Geometry: final body of the model. Coordinates: model frame, mm. A direction names the side the tool comes from. Give positions to 0.01 mm unless a question says otherwise; leave off trailing zeros. Write each loop counter-clockwise with the first axis right and the second up, starting at its lowest first coordinate (ties: lowest second). Pieces come first, ordered by that corner, then holes.
from build123d import *

# Parameters (mm, degrees)
SKETCH1_W                = 32
SKETCH1_H                = 28.5
BOSS_EXTRUDE1_DEPTH      = 8
BOSS_EXTRUDE2_DEPTH      = 28.5
SKETCH4_R                = 7.625
CUT_EXTRUDE2_DEPTH       = 26.5
SKETCH5_R                = 6
CUT_EXTRUDE3_DEPTH       = 39.581083448
CUT_EXTRUDE1_DEPTH       = 25.805493343
CUT_EXTRUDE1_DEPTH_BACK  = 25.805493343
SKETCH2_R                = 1.6
CUT_EXTRUDE4_DEPTH       = 25.805493451
CUT_EXTRUDE4_DEPTH_BACK  = 2.2
BOSS_EXTRUDE3_DEPTH      = 4
BOSS_EXTRUDE3_DEPTH_BACK = 4
SKETCH8_R                = 1.6
CUT_EXTRUDE5_DEPTH       = 42.764219136


with BuildPart() as part:
    # Sketch1 → Boss-Extrude1 (new body)
    with BuildSketch(Plane(origin=(0, 0, 0), x_dir=(1, 0, 0), z_dir=(0, 1, 0))):
        Rectangle(SKETCH1_W, SKETCH1_H)
    extrude(amount=BOSS_EXTRUDE1_DEPTH)

    # Sketch3 → Boss-Extrude2 (add, through all)
    with BuildSketch(Plane.XY.offset(14.25)):
        with BuildLine():
            Line((-7.158910532, 0), (7.158910532, 0))
            ThreePointArc((7.158910532, 0), (0, 20.5), (-7.158910532, 0))
        make_face()
    extrude(amount=-BOSS_EXTRUDE2_DEPTH)

    # Sketch4 → Cut-Extrude2 (cut)
    with BuildSketch(Plane.XY.offset(14.25)):
        with Locations((0, 9)):
            Circle(SKETCH4_R)
    extrude(amount=-CUT_EXTRUDE2_DEPTH, mode=Mode.SUBTRACT)

    # Sketch5 → Cut-Extrude3 (cut, through all)
    with BuildSketch(Plane(origin=(0, 0, -14.25), x_dir=(-1, 0, 0), z_dir=(0, 0, -1))):
        with Locations((0, 9)):
            Circle(SKETCH5_R)
    extrude(amount=-CUT_EXTRUDE3_DEPTH, mode=Mode.SUBTRACT)

    # Sketch2 → Cut-Extrude1 (cut, two sides: drawn at the far end of the back side and taken through both)
    with BuildSketch(Plane(origin=(0, 8, 0), x_dir=(1, 0, 0), z_dir=(0, 1, 0)).offset(-CUT_EXTRUDE1_DEPTH_BACK)):
        with Locations(Location((-12, 8, 0), (0, 0, 270))):
            Circle(SKETCH2_R)
        with Locations(Location((12, 8, 0), (0, 0, 250.139850489))):
            Circle(SKETCH2_R)
        with Locations(Location((12, -8, 0), (0, 0, 270))):
            Circle(SKETCH2_R)
        with Locations(Location((-12, -8, 0), (0, 0, 289.860135815))):
            Circle(SKETCH2_R)
    extrude(amount=CUT_EXTRUDE1_DEPTH + CUT_EXTRUDE1_DEPTH_BACK, mode=Mode.SUBTRACT)

    # Sketch6 → Cut-Extrude4 (cut, two sides: drawn at the far end of the back side and taken through both)
    with BuildSketch(Plane(origin=(0, 8, 0), x_dir=(1, 0, 0), z_dir=(0, 1, 0)).offset(-CUT_EXTRUDE4_DEPTH_BACK)):
        Polygon((-12, 11.464101615), (-15, 9.732050808), (-15, 6.267949192), (-12, 4.535898385), (-9, 6.267949192), (-9, 9.732050808), align=None)
        Polygon((-9, -9.732050808), (-12, -11.464101615), (-15, -9.732050808), (-15, -6.267949192), (-12, -4.535898385), (-9, -6.267949192), align=None)
        Polygon((12, -11.464101615), (15, -9.732050808), (15, -6.267949192), (12, -4.535898385), (9, -6.267949192), (9, -9.732050808), align=None)
        Polygon((9, 9.732050808), (12, 11.464101615), (15, 9.732050808), (15, 6.267949192), (12, 4.535898385), (9, 6.267949192), align=None)
    extrude(amount=CUT_EXTRUDE4_DEPTH + CUT_EXTRUDE4_DEPTH_BACK, mode=Mode.SUBTRACT)

    # Sketch8 → Boss-Extrude3 (add, two sides: drawn at the far end of the back side and taken through both)
    with BuildSketch(Plane(origin=(0, 0, 0), x_dir=(0, 0, -1), z_dir=(1, 0, 0)).offset(-BOSS_EXTRUDE3_DEPTH_BACK)):
        with BuildLine():
            Line((-3.5, 22.5), (-3.5, 18.5))
            Line((-3.5, 18.5), (3.5, 18.5))
            Line((3.5, 18.5), (3.5, 22.5))
            ThreePointArc((3.5, 22.5), (0, 26), (-3.5, 22.5))
        make_face()
        with Locations((0, 22.5)):
            Circle(SKETCH8_R, mode=Mode.SUBTRACT)
    extrude(amount=BOSS_EXTRUDE3_DEPTH + BOSS_EXTRUDE3_DEPTH_BACK)

    # Sketch9 → Cut-Extrude5 (cut, through all)
    with BuildSketch(Plane.XY.offset(14.25)):
        with BuildLine():
            Line((0, 9), (1.743114855, 28.923893962))
            ThreePointArc((1.743114855, 28.923893962), (0, 29), (-1.743114855, 28.923893962))
            Line((-1.743114855, 28.923893962), (0, 9))
        make_face()
    extrude(amount=-CUT_EXTRUDE5_DEPTH, mode=Mode.SUBTRACT)


solid = part.part
Q1. Section B-B on y = 13.25. Output: boundary loops of the cut face in (x, z), plus the area to 3 significant figures.
Filled sheet:
outline: (-10.69, -14.25) - (-4.24, -14.25) - (-4.24, -12.25) - (-6.33, -12.25) - (-6.33, 14.25) - (-10.69, 14.25) - (-10.69, 10.71) - (-9, 9.73) - (-9, 6.27) - (-10.69, 5.29) - (-10.69, -5.29) - (-9, -6.27) - (-9, -9.73) - (-10.69, -10.71) - close; (4.24, -14.25) - (10.69, -14.25) - (10.69, -10.71) - (9, -9.73) - (9, -6.27) - (10.69, -5.29) - (10.69, 5.29) - (9, 6.27) - (9, 9.73) - (10.69, 10.71) - (10.69, 14.25) - (6.33, 14.25) - (6.33, -12.25) - (4.24, -12.25) - close
area: 227 mm2
Q2. Section A-A on z = 0. Output: boundary loops of the cut face in (x, y) (3 decimals).
Filled sheet:
outline: (-16, 0) - (16, 0) - (16, 8) - (11.456, 8) arc R11.5 ccw to (4, 19.782) - (4, 20.9) - (1.041, 20.9) - (0.665, 16.596) arc R7.625 cw (long way) to (-0.665, 16.596) - (-1.041, 20.9) - (-4, 20.9) - (-4, 19.782) arc R11.5 ccw to (-11.456, 8) - (-16, 8) - close; (-4, 24.1) - (-1.321, 24.1) - (-1.487, 26) - (-4, 26) - close; (1.321, 24.1) - (4, 24.1) - (4, 26) - (1.487, 26) - close
Q3. Section C-C on y = 21.5. Output: boundary loops of the cut face in (x, z), plus the area to 3 significant figures.
Filled sheet:
outline: (-4, -3.5) - (-1.09, -3.5) - (-1.09, -1.25) - (-4, -1.25) - close; (-4, 1.25) - (-1.09, 1.25) - (-1.09, 3.5) - (-4, 3.5) - close; (1.09, -3.5) - (4, -3.5) - (4, -1.25) - (1.09, -1.25) - close; (1.09, 1.25) - (4, 1.25) - (4, 3.5) - (1.09, 3.5) - close
area: 26.2 mm2
Q4. Pull-direction query (Z, two-part tool) for faces 3 (the flat face through (13.5, 6.9, -5.4)), 4 (the cylindrical face through (-0.326, 1.382, 1.185)), 5 (the flat face through (10.146, 9.756, -10.394)), 6 (the flat face through (-3, 21, 3.5)); classes: released by +Z, released by -Z, zero draft, split by the parting line, or undercut.
Filled sheet:
face 3: undercut
face 4: zero draft
face 5: undercut
face 6: released by +Z
Q5. Pin query (flat end, axial travel): P1, Ø3, axis at y = 21.5, z = -1.5, coming from the -X side; P2, Ø5, axis at x = 12, z = -7.5, coming from the +Y side; P3, Ø1.4, axis at x = -12.5, z = 4, coming from the +Y side. Return the tip coordinate at first contact, or that it passes through.
Filled sheet:
P1: stops at x = -4
P2: stops at y = 5.8
P3: stops at y = 8
Q6. Access query for faces 1 (the flat face through (0, 0, 0)), 2 (the flat face through (10.146, 9.756, 10.394)). Directions: +Z, -Z, +X, -X, +Y, -Y. A direction counts if a zero-diameter tool reaches every point of the face in a straight line with its end or side. Return the directions, or none.
Filled sheet:
face 1: +Z, -Z, +X, -X, -Y
face 2: +Y
Q7. Section D-D on z = 3. Output: boundary loops of the cut face in (x, y) (3 decimals), plus the area to 3 significant figures.
Filled sheet:
outline: (-16, 0) - (16, 0) - (16, 8) - (11.456, 8) arc R11.5 ccw to (4, 19.782) - (4, 24.303) - (1.339, 24.303) - (0.665, 16.596) arc R7.625 cw (long way) to (-0.665, 16.596) - (-1.339, 24.303) - (-4, 24.303) - (-4, 19.782) arc R11.5 ccw to (-11.456, 8) - (-16, 8) - close
area: 321 mm2
Q8. Ray query, line 1 along Z through (x, y) = (-12, 4.6); line 2 along Z through (x, y) = (-14.5, 6.25); line 3 along X through (y, z) = (4, 7.5). Return the intervals inside material, ascending.
Filled sheet:
line 1: z = -14.25 to -9.6, -6.4 to 6.4, 9.6 to 14.25
line 2: z = -14.25 to -10.02, -5.98 to 5.98, 10.02 to 14.25
line 3: x = -16 to -13.52, -10.48 to -5.76, 5.76 to 10.48, 13.52 to 16
